Could you check a few things on this model? Use its own coordinates, in mm. Face numbers are marked on the shaded views. Give positions to 0.01 mm unless a question says otherwise; leave off trailing zeros. Loops run counter-clockwise (first coordinate to the right, second up) from the corner with the lowest first, then second, coordinate; pieces in that order, holes last. Notation, with made-up numbers: (74.5, 33) -> (81.5, 33) arc R23 cw to (81.5, 72) -> close; hole circle Ø1 at (-35.5, -17). An arc over 180 degrees is marked (long way). Put each result on its own line as item: value.
```python
from build123d import *

# Parameters (mm, degrees)
SKETCH_1_W          = 21
SKETCH_1_H          = 6
EXTRUDE_1_DEPTH     = 6
SKETCH_2_R          = 1.55
CUT_EXTRUDE_1_DEPTH = 6
SKETCH_3_R          = 1.55
CUT_EXTRUDE_2_DEPTH = 6


with BuildPart() as part:
    # 草图1 → 凸台-拉伸1 (new body)
    with BuildSketch(Plane(origin=(0, 0, 0), x_dir=(1, 0, 0), z_dir=(0, 1, 0))):
        Rectangle(SKETCH_1_W, SKETCH_1_H)
    extrude(amount=EXTRUDE_1_DEPTH)

    # 草图2 → 切除-拉伸1 (cut)
    with BuildSketch(Plane(origin=(0, 0, -3), x_dir=(-1, 0, 0), z_dir=(0, 0, -1))):
        with Locations((-7.875, 3)):
            Circle(SKETCH_2_R)
        with Locations((2.625, 3)):
            Circle(SKETCH_2_R)
    extrude(amount=-CUT_EXTRUDE_1_DEPTH, mode=Mode.SUBTRACT)

    # 草图3 → 切除-拉伸2 (cut)
    with BuildSketch(Plane.XZ):
        with Locations(Location((-7.875, 0, 0), (0, 0, 270))):
            Circle(SKETCH_3_R)
        with Locations(Location((2.625, 0, 0), (0, 0, 270))):
            Circle(SKETCH_3_R)
    extrude(amount=-CUT_EXTRUDE_2_DEPTH, mode=Mode.SUBTRACT)


solid = part.part
```
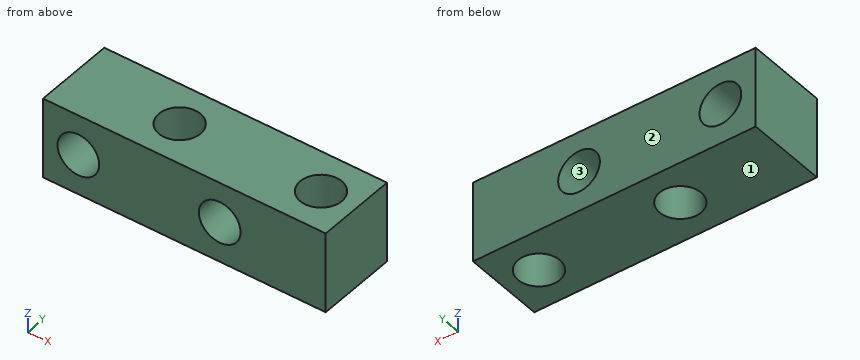
1. If we section it at B-B (y = 2.55): List the corners of the cut face in (x, z) for me (3 decimals), then the cut area to 3 significant figures.
Recorded:
outline: (-10.5, -3) -> (-4.108, -3) -> (-4.108, 3) -> (-10.5, 3) -> close; (-1.142, -3) -> (6.392, -3) -> (6.392, 3) -> (-1.142, 3) -> close; (9.358, -3) -> (10.5, -3) -> (10.5, 3) -> (9.358, 3) -> close; hole circle Ø3.1 at (-7.875, 0); hole circle Ø3.1 at (2.625, 0)
area: 75.3 mm^2
2. If we section it at C-C (z = -2.45): List the corners of the cut face in (x, y) for me (3 decimals).
Recorded:
outline: (-10.5, 0) -> (10.5, 0) -> (10.5, 6) -> (-10.5, 6) -> close; hole circle Ø3.1 at (-2.625, 3); hole circle Ø3.1 at (7.875, 3)
3. If we section it at D-D (x = 8.5): List the corners of the cut face in (y, z) for me, then the cut area to 3 significant figures.
Recorded:
outline: (0, -3) -> (1.58, -3) -> (1.58, 3) -> (0, 3) -> close; (4.42, -3) -> (6, -3) -> (6, 3) -> (4.42, 3) -> close
area: 19.0 mm^2
4. If we section it at A-A (z = 0): List the corners of the cut face in (x, y) for me (3 decimals).
Recorded:
outline: (-10.5, 0) -> (-9.425, 0) -> (-9.425, 6) -> (-10.5, 6) -> close; (-6.325, 0) -> (1.075, 0) -> (1.075, 6) -> (-6.325, 6) -> close; (4.175, 0) -> (10.5, 0) -> (10.5, 6) -> (4.175, 6) -> close; hole circle Ø3.1 at (-2.625, 3); hole circle Ø3.1 at (7.875, 3)
5. Thinking about a two-plate mould opening in Z: for the marked faces 1, 2 and 3, which applies, pulls with the +Z half, pulls with the -Z half, needs draft (parallel to the pull), parting line crosses it, or undercut?
Recorded:
face 1: pulls with the -Z half
face 2: needs draft
face 3: undercut
6. I need wall thicknesses on line 1 (X direction, y = 5.65, z = -0.6); line 2 (X direction, y = 2.4, z = -1.7); line 3 (X direction, y = 1.8, z = 0) (3 decimals). Which ranges of each line are inside material? Lowest first, please.
Recorded:
line 1: x = -10.5 to -9.3, -6.45 to 1.2, 4.05 to 10.5
line 2: x = -10.5 to -4.05, -1.2 to 6.45, 9.3 to 10.5
line 3: x = -10.5 to -9.425, -6.325 to -3.606, -1.644 to 1.075, 4.175 to 6.894, 8.856 to 10.5
